Here's how the part is built. I have some questions about the finished solid (model axes, mm). A direction names the side the tool comes from. Coordinates: 2 decimals unless noted, no trailing zeros. Order: outer loops, then holes, each group sorted by start corner. A loop starts at its lowest first (then second) coordinate and runs counter-clockwise, first axis right, second up. Notation, with made-up numbers: (-33, 34) -> (-24, 34) arc R26 ccw to (-24, 64) -> close; hole circle Ø9 at (-9.75, 81). An arc over 180 degrees is marked (long way). One line per item, written item: value. Start each with the question number.
```python
from build123d import *

# Parameters (mm, degrees)
EXTRUDE_1_DEPTH      = 30
SKETCH_2_R           = 44.45
CUT_EXTRUDE_1_DEPTH  = 4
SKETCH_3_R           = 25.5
SKETCH_3_R_2         = 2.25
CUT_EXTRUDE_2_DEPTH  = 188.619295383
CUT_EXTRUDE_3_DEPTH  = 189.215302247
SKETCH_5_R           = 1.65
CUT_EXTRUDE_4_DEPTH  = 189.215302247
EXTRUDE_START        = -30
EXTRUDE_2_DEPTH      = 30
CUT_EXTRUDE_5_DEPTH  = 198.040604952
CUT_EXTRUDE_7_DEPTH  = 233.432785983
CUT_EXTRUDE_8_DEPTH  = 233.432785983
CUT_EXTRUDE_9_DEPTH  = 233.432785983
FILLET_1_R           = 5
CUT_EXTRUDE_10_DEPTH = 233.432785983
EXTRUDE_START_2      = -5
EXTRUDE_3_DEPTH      = 5
EXTRUDE_4_DEPTH      = 5
SKETCH_14_R          = 4.25
CUT_EXTRUDE_11_DEPTH = 189.364728478
SKETCH_16_W          = 43
SKETCH_16_H          = 30
CUT_EXTRUDE_12_DEPTH = 233.432785983
EXTRUDE_7_REACH      = 188.592
SKETCH_18_W          = 210
SKETCH_18_H          = 5
EXTRUDE_8_DEPTH      = 210
EXTRUDE_9_DEPTH      = 5
EXTRUDE_10_DEPTH     = 5
SKETCH_22_R          = 4.25
CUT_EXTRUDE_13_DEPTH = 187.984035343
FILLET_2_R           = 5


with BuildPart() as part:
    # 草图1 → 凸台-拉伸1 (new body)
    with BuildSketch(Plane(origin=(0, 0, 0), x_dir=(1, 0, 0), z_dir=(0, 1, 0))):
        with BuildLine():
            Line((170, 31.93), (170, -31.93))
            ThreePointArc((170, -31.93), (167.781993847, -38.210172909), (162.111885646, -41.704453387))
            Line((162.111885646, -41.704453387), (15.839142344, -73.308400404))
            ThreePointArc((15.839142344, -73.308400404), (-75, 0), (15.839142344, 73.308400404))
            Line((15.839142344, 73.308400404), (162.111885646, 41.704453387))
            ThreePointArc((162.111885646, 41.704453387), (167.781993847, 38.210172909), (170, 31.93))
        make_face()
    extrude(amount=EXTRUDE_1_DEPTH)

    # 草图2 → 切除-拉伸1 (cut)
    with BuildSketch(Plane(origin=(0, 30, 0), x_dir=(1, 0, 0), z_dir=(0, 1, 0))):
        with Locations(Location((0, 0, 0), (0, 0, 270))):
            Circle(SKETCH_2_R)
    extrude(amount=-CUT_EXTRUDE_1_DEPTH, mode=Mode.SUBTRACT)

    # 草图3 → 切除-拉伸2 (cut, through all)
    with BuildSketch(Plane(origin=(0, 26, 0), x_dir=(1, 0, 0), z_dir=(0, 1, 0))):
        with Locations(Location((0, 0, 0), (0, 0, 270))):
            Circle(SKETCH_3_R)
        with Locations(Location((0, 41, 0), (0, 0, 270))):
            Circle(SKETCH_3_R_2)
        with Locations(Location((28.991378029, 28.991378029, 0), (0, 0, 270))):
            Circle(SKETCH_3_R_2)
        with Locations(Location((41, 0, 0), (0, 0, 270))):
            Circle(SKETCH_3_R_2)
        with Locations(Location((28.991378029, -28.991378029, 0), (0, 0, 270))):
            Circle(SKETCH_3_R_2)
        with Locations(Location((0, -41, 0), (0, 0, 270))):
            Circle(SKETCH_3_R_2)
        with Locations(Location((-28.991378029, -28.991378029, 0), (0, 0, 270))):
            Circle(SKETCH_3_R_2)
        with Locations(Location((-41, 0, 0), (0, 0, 270))):
            Circle(SKETCH_3_R_2)
        with Locations(Location((-28.991378029, 28.991378029, 0), (0, 0, 270))):
            Circle(SKETCH_3_R_2)
    extrude(amount=-CUT_EXTRUDE_2_DEPTH, mode=Mode.SUBTRACT)

    # 草图4 → 切除-拉伸3 (cut, through all)
    with BuildSketch(Plane(origin=(0, 30, 0), x_dir=(1, 0, 0), z_dir=(0, 1, 0))):
        with BuildLine():
            Line((124, 18.5), (134, 18.5))
            ThreePointArc((134, 18.5), (152.5, 0), (134, -18.5))
            Line((134, -18.5), (124, -18.5))
            ThreePointArc((124, -18.5), (105.5, 0), (124, 18.5))
        make_face()
    extrude(amount=-CUT_EXTRUDE_3_DEPTH, mode=Mode.SUBTRACT)

    # 草图5 → 切除-拉伸4 (cut, through all)
    with BuildSketch(Plane(origin=(0, 30, 0), x_dir=(1, 0, 0), z_dir=(0, 1, 0))):
        with Locations(Location((116.75, 25.5, 0), (0, 0, 270))):
            Circle(SKETCH_5_R)
        with Locations(Location((141.25, 25.5, 0), (0, 0, 270))):
            Circle(SKETCH_5_R)
        with Locations(Location((141.25, -25.5, 0), (0, 0, 270))):
            Circle(SKETCH_5_R)
        with Locations(Location((116.75, -25.5, 0), (0, 0, 270))):
            Circle(SKETCH_5_R)
    extrude(amount=-CUT_EXTRUDE_4_DEPTH, mode=Mode.SUBTRACT)

    # 草图6 → 凸台-拉伸2 (add)
    with BuildSketch(Plane(origin=(0, 30, 0), x_dir=(1, 0, 0), z_dir=(0, 1, 0)).offset(EXTRUDE_START)):
        with BuildLine():
            Line((158, 95), (-52, 95))
            Line((-52, 95), (-52, 54.046276467))
            ThreePointArc((-52, 54.046276467), (-20.48558667, 72.148047366), (15.839142344, 73.308400404))
            Line((15.839142344, 73.308400404), (158, 42.592874655))
            Line((158, 42.592874655), (158, 95))
        make_face()
        with BuildLine():
            ThreePointArc((15.839142344, -73.308400404), (-20.48558667, -72.148047366), (-52, -54.046276467))
            Line((-52, -54.046276467), (-52, -95))
            Line((-52, -95), (158, -95))
            Line((158, -95), (158, -42.592874655))
            Line((158, -42.592874655), (15.839142344, -73.308400404))
        make_face()
    extrude(amount=EXTRUDE_2_DEPTH)

    # 草图7 → 切除-拉伸5 (cut, through all)
    with BuildSketch(Plane(origin=(0, 30, 0), x_dir=(1, 0, 0), z_dir=(0, 1, 0))):
        with BuildLine():
            Line((-52, 54.046276467), (-52, -54.046276467))
            ThreePointArc((-52, -54.046276467), (-75, 0), (-52, 54.046276467))
        make_face()
        with BuildLine():
            Line((158, 42.592874655), (158, -42.592874655))
            Line((158, -42.592874655), (162.111885646, -41.704453387))
            ThreePointArc((162.111885646, -41.704453387), (167.781993847, -38.210172909), (170, -31.93))
            Line((170, -31.93), (170, 31.93))
            ThreePointArc((170, 31.93), (167.781993847, 38.210172909), (162.111885646, 41.704453387))
            Line((162.111885646, 41.704453387), (158, 42.592874655))
        make_face()
    extrude(amount=-CUT_EXTRUDE_5_DEPTH, mode=Mode.SUBTRACT)

    # 草图9 → 切除-拉伸7 (cut, through all)
    with BuildSketch(Plane.ZY.offset(52)):
        Polygon((-95, 20), (-60, 10.621778265), (-60, 30), (-95, 30), align=None)
    extrude(amount=-CUT_EXTRUDE_7_DEPTH, mode=Mode.SUBTRACT)

    # 草图10 → 切除-拉伸8 (cut, through all)
    with BuildSketch(Plane.ZY.offset(52)):
        Polygon((-95, 12.753066737), (-52, 1.231251463), (-52, 0), (-95, 0), align=None)
    extrude(amount=-CUT_EXTRUDE_8_DEPTH, mode=Mode.SUBTRACT)

    # 草图8 → 切除-拉伸9 (cut, through all)
    with BuildSketch(Plane.ZY.offset(52)):
        Polygon((0, 0), (52, 0), (52, 17.3), (-52, 17.3), (-52, 0), align=None)
    extrude(amount=-CUT_EXTRUDE_9_DEPTH, mode=Mode.SUBTRACT)

    # 圆角1
    fillet_1_edges = [part.edges().sort_by_distance(p)[0] for p in [
        (53, 10.621778265, -60),
    ]]
    fillet(fillet_1_edges, radius=FILLET_1_R)

    # 草图11 → 切除-拉伸10 (cut, through all)
    with BuildSketch(Plane.ZY.offset(52)):
        Polygon((-95, 12.753066737), (-93.188266684, 19.514547521), (-95, 20), align=None)
    extrude(amount=-CUT_EXTRUDE_10_DEPTH, mode=Mode.SUBTRACT)

    # 草图12 → 凸台-拉伸3 (add)
    with BuildSketch(Plane.ZY.offset(52).offset(EXTRUDE_START_2)):
        with BuildLine():
            Line((-93.188266684, 19.514547521), (-60, 30))
            Line((-60, 30), (-60, 17.137905129))
            ThreePointArc((-60, 17.137905129), (-61.956192855, 13.171138428), (-66.294095226, 12.308275998))
            Line((-66.294095226, 12.308275998), (-93.188266684, 19.514547521))
        make_face()
    extrude(amount=EXTRUDE_3_DEPTH)

    # 草图13 → 凸台-拉伸4 (add)
    with BuildSketch(Plane(origin=(158, 0, 0), x_dir=(0, 0, -1), z_dir=(1, 0, 0))):
        with BuildLine():
            Line((66.294095226, 12.308275998), (93.188266684, 19.514547521))
            Line((93.188266684, 19.514547521), (60, 30))
            Line((60, 30), (60, 17.137905129))
            ThreePointArc((60, 17.137905129), (61.956192855, 13.171138428), (66.294095226, 12.308275998))
        make_face()
    extrude(amount=-EXTRUDE_4_DEPTH)

    # 草图14 → 切除-拉伸11 (cut, through all)
    with BuildSketch(Plane(origin=(0, -5.089745962, -1.36379332), x_dir=(1, 0, 0), z_dir=(0, 0.9659258262890681, 0.2588190451025214))):
        with Locations(Location((-27, 82.063690052, 0), (0, 0, 270))):
            Circle(SKETCH_14_R)
        with Locations(Location((23, 82.063690052, 0), (0, 0, 270))):
            Circle(SKETCH_14_R)
        with Locations(Location((83, 82.063690052, 0), (0, 0, 270))):
            Circle(SKETCH_14_R)
        with Locations(Location((133, 82.063690052, 0), (0, 0, 270))):
            Circle(SKETCH_14_R)
    extrude(amount=-CUT_EXTRUDE_11_DEPTH, mode=Mode.SUBTRACT)

    # 草图16 → 切除-拉伸12 (cut, through all)
    with BuildSketch(Plane.ZY.offset(52)):
        with Locations((73.5, 15)):
            Rectangle(SKETCH_16_W, SKETCH_16_H)
    extrude(amount=-CUT_EXTRUDE_12_DEPTH, mode=Mode.SUBTRACT)

    # 凸台-拉伸7: up to this plane
    extrude_7_end = Plane(origin=(0, -11.851226746, -3.175526636), z_dir=(0, -0.9659258262890681, -0.25881904510252146))
    # 草图18 → 凸台-拉伸7 (add, up to the surface)
    with BuildSketch(Plane(origin=(0, 30, 0), x_dir=(1, 0, 0), z_dir=(0, 1, 0)), mode=Mode.PRIVATE) as extrude_7_sk1:
        with Locations((53, -54.5)):
            Rectangle(SKETCH_18_W, SKETCH_18_H)
    extrude_7_tool1 = split(extrude(extrude_7_sk1.sketch, amount=-EXTRUDE_7_REACH, mode=Mode.PRIVATE), bisect_by=extrude_7_end, keep=Keep.BOTH, mode=Mode.PRIVATE)
    add(extrude_7_tool1.solids().sort_by_distance((53, 30, 54.5))[0])

    # 草图19 → 凸台-拉伸8 (add)
    with BuildSketch(Plane.ZY.offset(52)):
        Polygon((57, -27.975210512), (90.188266684, -36.867979769), (92, -30.106498985), (57, -20.72827725), align=None)
    extrude(amount=-EXTRUDE_8_DEPTH)

    # 草图20 → 凸台-拉伸9 (add)
    with BuildSketch(Plane.ZY.offset(52)):
        Polygon((92, -30.106498985), (57, -20.72827725), (57, 30), align=None)
    extrude(amount=-EXTRUDE_9_DEPTH)

    # 草图21 → 凸台-拉伸10 (add)
    with BuildSketch(Plane(origin=(158, 0, 0), x_dir=(0, 0, -1), z_dir=(1, 0, 0))):
        Polygon((-57, 30), (-92, -30.106498985), (-57, -20.72827725), align=None)
    extrude(amount=-EXTRUDE_10_DEPTH)

    # 草图22 → 切除-拉伸13 (cut, through all)
    with BuildSketch(Plane(origin=(0, -5.089745962, -1.36379332), x_dir=(1, 0, 0), z_dir=(0, 0.9659258262890686, 0.25881904510251946))):
        with Locations(Location((-27, -77.936309948, 0), (0, 0, 270))):
            Circle(SKETCH_22_R)
        with Locations(Location((23, -69.936309948, 0), (0, 0, 270))):
            Circle(SKETCH_22_R)
        with Locations(Location((83, -69.936309948, 0), (0, 0, 270))):
            Circle(SKETCH_22_R)
        with Locations(Location((133, -77.936309948, 0), (0, 0, 270))):
            Circle(SKETCH_22_R)
    extrude(amount=-CUT_EXTRUDE_13_DEPTH, mode=Mode.SUBTRACT)

    # 圆角2
    fillet_2_edges = [part.edges().sort_by_distance(p)[0] for p in [
        (53, -20.72827725, 57),
    ]]
    fillet(fillet_2_edges, radius=FILLET_2_R)


solid = part.part
```
Q1. Imagine slicing it at A-A (z = 13). Write out the boundary of the cut face in (x, y).
Q2. For faces 1 (the face through (105.504, 23.739, 0.407)), 2 (the face through (153, -6, 67)), 3 (the face through (51.6, 15.96, -79.93)), which set-ups out of +Z, -Z, +X, -X, +Y, -Y let a thin tool reach every point of the face, with its end or its side?
Q3. For P1, Ø11, axis at x = 128, y = 21.5, coming from the -Z side; P2, Ø6, axis at x = 0.5, z = -25, coming from the +Y side; P3, Ø2.5, axis at x = 141.25, z = -25.5, coming from the +Y side; P4, Ø4, axis at x = 116.75, z = -25.5, coming from the -Y side, each with a flat end and sliding along its axis, tell me the tip position at first contact or that it passes through.
Q4. If we mould it in two halves opening along Z, with no side actions, what happens to faces 4 (the face through (51.53, 7.073, -73.801)), 5 (the face through (54.4, -19.899, 58.006)), 6 (the face through (52, 30, -2)), 7 (the face through (137.214, -28.451, 72.489))? For each: +Z half, -Z half, draft (parallel to the pull), parting line (faces both ways), or undercut.
Q5. Imagine slicing it at B-B (y = 5). Write out the boundary of the cut face in (x, z).
Q6. I need wall thicknesses on line 1 (X direction, y = 28.2, z = 0); line 2 (X direction, y = 23, z = 0); line 3 (Z direction, x = 54.5, y = 27). Which ranges of each line are inside material? Lowest first, please.
Q7. Imagine slicing it at D-D (x = -12). Write out the boundary of the cut face in (y, z), plus the area to 3 significant figures.
Q8. Imagine slicing it at C-C (x = 13). Write out the boundary of the cut face in (y, z).
Completed:
1. outline: (-52, 17.3) -> (-21.94, 17.3) -> (-21.94, 26) -> (-42.51, 26) -> (-42.51, 30) -> (-52, 30) -> close; (21.94, 17.3) -> (110.84, 17.3) -> (110.84, 30) -> (42.51, 30) -> (42.51, 26) -> (21.94, 26) -> close; (147.16, 17.3) -> (158, 17.3) -> (158, 30) -> (147.16, 30) -> close
2. face 1: +Y, -Y
2. face 2: +Z, +Y
2. face 3: +Y
3. P1: stops at z = -94.13
3. P2: stops at y = 26
3. P3: passes through
3. P4: stops at y = 17.3
4. face 4: -Z half
4. face 5: +Z half
4. face 6: draft
4. face 7: undercut
5. outline: (-52, -66.07) -> (158, -66.07) -> (158, -52) -> (-52, -52) -> close; (-52, 52) -> (158, 52) -> (158, 71.56) -> (153, 71.56) -> (153, 57) -> (-47, 57) -> (-47, 71.56) -> (-52, 71.56) -> close
6. line 1: x = -52 to -44.45, 44.45 to 105.5, 152.5 to 158
6. line 2: x = -52 to -43.25, -38.75 to -25.5, 25.5 to 38.75, 43.25 to 105.5, 152.5 to 158
6. line 3: z = -60 to 57
7. outline: (-36.87, 90.19) -> (-26.64, 52) -> (17.3, 52) -> (17.3, 22.5) -> (26, 22.5) -> (26, 42.8) -> (30, 42.8) -> (30, 57) -> (-16.89, 57) arc R5 cw to (-21.72, 60.71) -> (-30.11, 92) -> close; (1.23, -52) -> (12.75, -95) -> (19.51, -93.19) -> (12.31, -66.29) arc R5 cw to (17.14, -60) -> (30, -60) -> (30, -42.8) -> (26, -42.8) -> (26, -22.5) -> (17.3, -22.5) -> (17.3, -52) -> close
7. area: 1,600 mm2
8. outline: (-36.87, 90.19) -> (-26.64, 52) -> (17.3, 52) -> (17.3, 21.94) -> (26, 21.94) -> (26, 42.51) -> (30, 42.51) -> (30, 57) -> (-16.89, 57) arc R5 cw to (-21.72, 60.71) -> (-30.11, 92) -> close; (1.23, -52) -> (12.75, -95) -> (19.51, -93.19) -> (12.31, -66.29) arc R5 cw to (17.14, -60) -> (30, -60) -> (30, -42.51) -> (26, -42.51) -> (26, -21.94) -> (17.3, -21.94) -> (17.3, -52) -> close
